from build123d import *

# Parameters (mm, degrees)
F0_W     = 1905
F0_H     = 635
F1_DEPTH = 127
F2_R     = 317.5
F3_DEPTH = 127
F4_DEPTH = 127
F5_DEPTH = 508
F6_R     = 254
F7_DEPTH = 635
F9_DEPTH = 254.001


with BuildPart() as f1:
    # F0 (on Top) → F1 (new body, symmetric)
    with BuildSketch(Plane.XY):
        with Locations((177.6640671305, 114.6936982827)):
            Rectangle(F0_W, F0_H)
    extrude(amount=F1_DEPTH, both=True)

    # F2 (on face) → F3 (join, symmetric)
    with BuildSketch(Plane.XY.offset(127)):
        with Locations((-774.8359328695, 114.6936982827)):
            Circle(F2_R)
    extrude(amount=F3_DEPTH, both=True)

    # F4 (add): a face of the model
    f4_faces = [f1.faces().sort_by_distance(p)[0] for p in [
        (-909.5871180206, 114.6936982827, 0),
    ]]
    extrude(f4_faces, amount=F4_DEPTH)

    # F5 (add): a face of the model
    f5_faces = [f1.faces().sort_by_distance(p)[0] for p in [
        (-774.8359328695, 114.6936982827, 254),
    ]]
    extrude(f5_faces, amount=F5_DEPTH)

    # F6 (on face) → F7 (cut)
    with BuildSketch(Plane.XY.offset(762)):
        with Locations((-774.8359328695, 114.6936982827)):
            Circle(F6_R)
    extrude(amount=-F7_DEPTH, mode=Mode.SUBTRACT)

    # F8 (on face) → F9 (cut, through all)
    with BuildSketch(Plane.XY.offset(127)):
        with BuildLine():
            Line((1130.1640671305, 281.3425958157), (183.8743803286, 312.780909445))
            ThreePointArc((183.8743803286, 312.780909445), (-9.3430063716, 128.9567688771), (177.6640671305, -61.1816744713))
            Line((177.6640671305, -61.1816744713), (1130.1640671305, -61.1816744713))
            Line((1130.1640671305, -61.1816744713), (1130.1640671305, 281.3425958157))
        make_face()
    extrude(amount=-F9_DEPTH, mode=Mode.SUBTRACT)


solid = f1.part
Can you work these out from the model? Positions are in its coordinate system, mm. A direction names the side the tool comes from. Coordinates: 2 decimals unless noted, no trailing zeros. Loops run counter-clockwise (first coordinate to the right, second up) from the corner with the lowest first, then second, coordinate; pieces in that order, holes last. Notation, with made-up numbers: M 69,-1.5 L 100,-1.5 A4 cw 100,5.5 Z; hole C 30.5,-25.5 d11. An arc over 180 degrees is marked long. Return JSON: item names as keys, results as strings. Group by question number.
Item 1: I'm going to push flat-ended pins straight in: pin 1 Ø2 at (x, y) = (-258.5, 80.5) entering from +Z; pin 2 Ø5 at (y, z) = (333.5, 103.5) entering from -X; pin 3 Ø6 at (y, z) = (332.5, 137) entering from -X. Where does each tip first touch, or does it pass through?
Item 2: Thinking about a two-plate mould opening in X: for faces 4 (the cylindrical face through (-9.228, 133.112, 1.778)), 5 (the flat face through (1130.164, 356, 2)), 6 (the flat face through (-244, 119, -127)), 7 (the cylindrical face through (-1028.59, 125.86, 448.94)), which applies, released by +X, released by -X, zero draft, split by the parting line, or undercut?
Item 3: Imagine slicing it at D-D (x = 258). Please give me the cut outline in (y, z).
Item 4: Imagine slicing it at C-C (y = 153). Please give me the cut outline in (x, z), and give its area (3 significant figures).
Item 5: Imagine slicing it at A-A (x = 956.5). Please give me the cut outline in (y, z).
Item 6: On a 3-axis mill with a long thin cutter (end or side, diameter ignored), from which of +Z, -Z, +X, -X, +Y, -Y can I reach the whole of each face in a straight line? I mean faces 1 (the flat face through (164, -202.806, 2)), 2 (the flat face through (-778, 118, 127)), 3 (the flat face through (647, -61.182, 2)). Say none if no direction works.
Item 7: Imagine slicing it at B-B (z = 49). Please give me the cut outline in (x, y), and give its area (3 significant figures).
Item 8: If I drill on L1, parallel to Z at x = -83.5, y = 134; L2, parallel to X at y = 111, z = 716; L3, parallel to X at y = 276.5, z = 626.5, over which ranges is the centre line in solid material (lowest first)? Write a range as from..to.
Verdict:
{
 "1": {"pin 1": "stops at z = 127", "pin 2": "stops at x = -1007.25", "pin 3": "stops at x = -1008.64"},
 "2": {"face 4": "undercut", "face 5": "released by +X", "face 6": "zero draft", "face 7": "undercut"},
 "3": {"outline": "M -202.81,-127 L -61.18,-127 L -61.18,127 L -202.81,127 Z; M 310.32,-127 L 432.19,-127 L 432.19,127 L 310.32,127 Z"},
 "4": {"outline": "M -1090.02,-127 L -7.39,-127 L -7.39,127 L -459.66,127 L -459.66,762 L -523.74,762 L -523.74,127 L -1025.93,127 L -1025.93,762 L -1090.02,762 Z", "area": "356,000 mm^2"},
 "5": {"outline": "M -202.81,-127 L -61.18,-127 L -61.18,127 L -202.81,127 Z; M 287.11,-127 L 432.19,-127 L 432.19,127 L 287.11,127 Z"},
 "6": {"face 1": "+Z, -Z, +X, -X, -Y", "face 2": "+Z", "face 3": "+Z, -Z, +X"},
 "7": {"outline": "M -774.84,-202.81 L 1130.16,-202.81 L 1130.16,-61.18 L 177.66,-61.18 A187.03 cw long 183.87,312.78 L 1130.16,281.34 L 1130.16,432.19 L -774.84,432.19 A317.5 ccw Z", "area": "972,000 mm^2"},
 "8": {"L1": "z = -127..127", "L2": "x = -1092.31..-1028.81, -520.86..-457.36", "L3": "x = -1048.01..-970.63, -579.04..-501.66"}
}
